Autodesk Inventor part; units mm, degrees
ref_plane "Work Plane2" through (0, 0, 7) normal (0, 0, 1) x (1, 0, 0)
ref_plane "Work Plane3" through (0, 0, 2) normal (0, 0, -1) x (-1, 0, 0)
ref_plane "YZ Plane" through (0, 0, 0) normal (1, 0, 0) x (0, 1, 0)
sketch "Sketch1" plane through (0, 0, 0) normal (0, 0, 1) x (1, 0, 0)
  circle A0 centre (0, 0) radius 10
  dimension "d0" = 20
extrude "Extrusion1" add sketch "Sketch1" along normal blind 2
sketch "Sketch2" plane through (0, 0, 2) normal (0, 0, 1) x (1, 0, 0)
  circle A0 centre (0, 0) radius 3.75
  dimension "d3" = 7.5
extrude "Extrusion2" add sketch "Sketch2" along normal blind 15
ref_plane "Work Plane2" through (0, 0, 7) normal (0, 0, 1) x (1, 0, 0)
sketch "Sketch7" plane through (0, 0, 7) normal (0, 0, 1) x (1, 0, 0)
  circle A0 centre (0, 0) radius 3.75
  circle A1 centre (0, 0) radius 5.75
  dimension "d27" = 2
extrude "Extrusion7" add sketch "Sketch7" against normal blind 2
sketch "Sketch8" plane through (0, 0, 5) normal (0, 0, -1) x (-1, 0, 0)
  circle A0 centre (0, 0) radius 5.75
  circle A1 centre (0, 0) radius 3.75
  circle A2 centre (0, 0) radius 5.75 construction
  line L0 (5.75, 0) -> (-5.75, 0) construction
  line L1 (-3.75, 0) -> (3.75, 0)
  line L2 (3.75, 0) -> (3.75, -18.3333)
  line L3 (3.75, -18.3333) -> (-3.75, -18.3333)
  line L4 (-3.75, -18.3333) -> (-3.75, 0)
  dimension "d31" = 18.3333
extrude "Extrusion8" add sketch "Sketch8" along normal blind 3 contours L4 A1 L2 A0 | A0 L2 L3 L4 picked at (2.8343, -4.1874)
sketch "Sketch9" plane through (0, 0, 2) normal (0, 0, -1) x (-1, 0, 0)
  arc A0 (-3.75, -4.3589) -> (3.75, -4.3589) centre (0, 0) ccw
  line L0 (3.75, -18.3333) -> (3.75, -4.3589)
  line L1 (-3.75, -18.3333) -> (3.75, -18.3333)
  line L2 (-3.75, -4.3589) -> (-3.75, -18.3333)
  line L3 (-2, -8) -> (2, -8)
  line L4 (2, -8) -> (2, -16)
  line L5 (2, -16) -> (-2, -16)
  line L6 (-2, -16) -> (-2, -8)
  dimension "d34" = 2
  dimension "d35" = 4
  dimension "d36" = 8
  dimension "d37" = 8
extrude "Extrusion9" cut sketch "Sketch9" against normal up to surface (3 mm away) draft 2 contours L3 L4 L5 L6
fillet "Fillet2" radius 0.25 4 edges at (0, -16.1048, 5) (2.1048, -12, 5) (-2.1048, -12, 5) (0, -7.8952, 5)
ref_plane "Work Plane3" through (0, 0, 2) normal (0, 0, -1) x (-1, 0, 0)
split "Split1" plane through (0, 0, 2) removes the side toward (0, 0, -1)
equation "\"d1\" = IG_gearThickness"
equation "\"d3\" = IG_shaftDiameter"
equation "\"d4\" = IG_shaftLength"
equation "\"Wheel_Related_W_\" = 0"
equation "\"W_innerDepth\" = 4"
equation "\"W_wallThickness\" = 2"
equation "\"W_holesClearance\" = 0.3"
equation "\"W_outerGearHoleDiameter\" = 5.3"
equation "\"W_innerGearHoleDiameter\" = 10.1"
equation "\"TempSpotReserved7\" = 0"
equation "\"TempSpotReserved8\" = 0"
equation "\"TempSpotReserved9\" = 0"
equation "\"TempSpotReserved10\" = 0"
equation "\"TempSpotReserved11\" = 0"
equation "\"TempSpotReserved12\" = 0"
equation "\"TempSpotReserved13\" = 0"
equation "\"TempSpotReserved14\" = 0"
equation "\"TempSpotReserved15\" = 0"
equation "\"TempSpotReserved16\" = 0"
equation "\"TempSpotReserved17\" = 0"
equation "\"TempSpotReserved18\" = 0"
equation "\"TempSpotReserved19\" = 0"
equation "\"TempSpotReserved20\" = 0"
equation "\"Inner_Gear_Related_IG_\" = 0"
equation "\"IG_shaftDiameter\" = 7.5"
equation "\"IG_shaftLength\" = 15"
equation "\"IG_gearThickness\" = 2"
equation "\"TempSpotReserved25\" = 0"
equation "\"TempSpotReserved26\" = 0"
equation "\"TempSpotReserved27\" = 0"
equation "\"TempSpotReserved28\" = 0"
equation "\"TempSpotReserved29\" = 0"
equation "\"TempSpotReserved30\" = 0"
equation "\"TempSpotReserved31\" = 0"
equation "\"TempSpotReserved32\" = 0"
equation "\"TempSpotReserved33\" = 0"
equation "\"TempSpotReserved34\" = 0"
equation "\"TempSpotReserved35\" = 0"
equation "\"TempSpotReserved36\" = 0"
equation "\"TempSpotReserved37\" = 0"
equation "\"TempSpotReserved38\" = 0"
equation "\"TempSpotReserved39\" = 0"
equation "\"TempSpotReserved40\" = 0"
equation "\"Outer_Gear_Related_OG_\" = 0"
equation "\"OG_distanceFromCenter\" = 23.33333"
equation "\"OG_shaftDiameter\" = 5"
equation "\"OG_gearDiameter\" = 26.66667"
equation "\"OG_shaftLength\" = 7"
equation "\"OG_gearThickness\" = 2"
equation "\"TempSpotReserved47\" = 0"
equation "\"TempSpotReserved48\" = 0"
equation "\"TempSpotReserved49\" = 0"
equation "\"TempSpotReserved50\" = 0"
equation "\"TempSpotReserved51\" = 0"
equation "\"TempSpotReserved52\" = 0"
equation "\"TempSpotReserved53\" = 0"
equation "\"TempSpotReserved54\" = 0"
equation "\"TempSpotReserved55\" = 0"
equation "\"TempSpotReserved56\" = 0"
equation "\"TempSpotReserved57\" = 0"
equation "\"TempSpotReserved58\" = 0"
equation "\"TempSpotReserved59\" = 0"
equation "\"TempSpotReserved60\" = 0"
equation "\"Leg_Extensions_Related_LE_\" = 0"
equation "\"LE_baseDiameter\" = 5"
equation "\"LE_maxLength\" = 24.6522"
equation "\"LE_thickness\" = 2.5"
equation "\"IG_ratioToOuterGear\" = 0.75"
equation "\"B_bearingThickness\" = 1"
equation "\"TempSpotReserved43\" = 0"
equation "\"TempSpotReserved45\" = 0"
equation "\"Thisisatest\" = 25.4"
equation "\"TempSpotReserved46\" = 0"
equation "\"TempSpotReserved44\" = 0"
equation "\"LE_offsetAboveOuterGear\" = 0"
equation "\"Bearing_Related_B_\" = 0"
equation "\"TempSpotReserved42\" = 0"
equation "\"OG_skirtOffset\" = 1"
equation "\"OG_skirtThickness\" = 1"
equation "\"IG_skirtThickness\" = 2"
equation "\"IG_extentionLength\" = 18.33333"
equation "\"IG_extentionThickness\" = 3"
equation "\"IG_slitWidth\" = 4"
equation "\"IG_slitlength\" = 8"
equation "\"IG_slitDistanceFromCenterHole\" = 8"
equation "\"IG_slitClearance\" = 0.2"
equation "\"Reserved_10\" = 0"
equation "\"Reserved_9\" = 0"
equation "\"Reserved_11\" = 0"
equation "\"Reserved_12\" = 0"
equation "\"Reserved_8\" = 0"
equation "\"Reserved_7\" = 0"
equation "\"Reserved_26\" = 0"
equation "\"Reserved_20\" = 0"
equation "\"Reserved_22\" = 0"
equation "\"Reserved_23\" = 0"
equation "\"Reserved_25\" = 0"
equation "\"Reserved_24\" = 0"
equation "\"Reserved_21\" = 0"
equation "\"Reserved_19\" = 0"
equation "\"Reserved_27\" = 0"
equation "\"Reserved_14\" = 0"
equation "\"Reserved_15\" = 0"
equation "\"Reserved_16\" = 0"
equation "\"Reserved_13\" = 0"
equation "\"Reserved_17\" = 0"
equation "\"Reserved_18\" = 0"
equation "\"Bearing_Related_BR_\" = 0"
equation "\"BR_bearingThickness\" = 1"
equation "\"Block_Related_BL_\" = 0"
equation "\"BL_width\" = 3.8"
equation "\"BL_length\" = 7.8"
equation "\"W_filletRadius\" = 0.25"
equation "\"W_extrutsionTaperAngle\" = 2deg"
equation "\"OG_protrudeDistance\" = 3"
properties part number "innerGear1"
Here's how the part is built. I have some questions about the finished solid (model axes, mm). A direction names the side the tool comes from. Round coordinates to 2 decimals unless told otherwise and drop trailing zeros. Order: outer loops, then holes, each group sorted by start corner. A loop starts at its lowest first (then second) coordinate and runs counter-clockwise, first axis right, second up. Notation, with made-up numbers: M 37.25,46.25 L 95.25,46.25 A22 cw 95.25,62.25 Z; hole C 37,-27 d7. An arc over 180 degrees is marked long. One line per question, with ' | ' between items.
1) For pin 1 Ø5 at (x, z) = (2, 13) entering from -Y; pin 2 Ø1 at (x, y) = (-2, -5.5) entering from +Z; pin 3 Ø0.9 at (y, z) = (-6, 3) entering from -X, each with a flat end and sliding along its axis, tell me the tip position at first contact or that it passes through.
Working result:
pin 1: y = -3.75 | pin 2: z = 7 | pin 3: x = -3.75
2) I want a section at A-A, the plane y = -12. Write out the boundary of the cut face in (x, z), then the cut area to 3 significant figures.
Working result:
outline: M -3.75,2 L -2,2 L -2.1,4.76 A0.25 ccw -2.35,5 L -3.75,5 Z; M 2,2 L 3.75,2 L 3.75,5 L 2.35,5 A0.25 ccw 2.1,4.76 Z | area: 10.2 mm²
3) I want a section at D-D, the plane y = 3. Write out the boundary of the cut face in (x, z).
Working result:
outline: M -4.91,5 L -2.25,5 L -2.25,2 L 2.25,2 L 2.25,5 L 4.91,5 L 4.91,7 L 2.25,7 L 2.25,17 L -2.25,17 L -2.25,7 L -4.91,7 Z
4) I need wall thicknesses on line 1 along Y through (x, z) = (0, 13.75); line 2 along Z through (x, y) = (-1.25, -16.5); line 3 along Z through (x, y) = (5.25, -1). Which ranges of each line are inside material? Lowest first, please.
Working result:
line 1: -3.75 to 3.75 | line 2: 2 to 5 | line 3: 5 to 7
5) I want a section at B-B, the plane x = 0. Write out the boundary of the cut face in (y, z).
Working result:
outline: M -18.33,2 L -16,2 L -16.1,4.76 A0.25 ccw -16.35,5 L -18.33,5 Z; M -8,2 L 3.75,2 L 3.75,5 L 5.75,5 L 5.75,7 L 3.75,7 L 3.75,17 L -3.75,17 L -3.75,7 L -5.75,7 L -5.75,5 L -7.65,5 A0.25 ccw -7.9,4.76 Z
6) I want a section at C-C, the plane z = 3.5. Write out the boundary of the cut face in (x, y).
Working result:
outline: M -3.75,-18.33 L 3.75,-18.33 L 3.75,0 A3.75 ccw -3.75,0 Z; hole M -2.05,-16.05 L 2.05,-16.05 L 2.05,-7.95 L -2.05,-7.95 Z
7) For faces 1 (the face through (-3.75, -9, 4)), 2 (the face through (3.75, -9, 4)), 3 (the face through (-0.08, 3.75, 3.48)), 4 (the face through (-3.746, -0.165, 11.93)), 5 (the face through (0, -18.333, 4)), which set-ups out of +Z, -Z, +X, -X, +Y, -Y let a thin tool reach every point of the face, with its end or its side?
Working result:
face 1: -Z, -X, +Y, -Y | face 2: -Z, +X, +Y, -Y | face 3: -Z, +Y | face 4: +Z | face 5: +Z, -Z, +X, -X, -Y
